Check sheet for the modelled part. Datum: model origin and axes. Units: mm. A direction names the side the tool comes from. Give positions to 0.01 mm unless a question says otherwise; leave off trailing zeros. Write each loop counter-clockwise with the first axis right and the second up, starting at its lowest first coordinate (ties: lowest second). Pieces come first, ordered by that corner, then holes. Notation, with made-up numbers: M 80,8 L 96,8 A16 cw 96,18 Z; hole C 27,4 d8. An arc over 180 degrees is marked long. Use CSV: the item, a comma, the result in double quotes. Start each with the question number.
1. Scan lines: line 1 (Z direction, x = 152.5, y = -0.55); line 2 (Z direction, x = -189.5, y = -0.05); line 3 (X direction, y = -1.05, z = 150.5). Record each from-to range of solid material in increasing order.
2. Access from +Z, -Z, +X, -X, +Y, -Y to the whole of each face (thin tool, end or side, straight path). Record for faces 4 (the face through (311.773, -1.014, 21.597)), 5 (the face through (321.043, -0.986, 13.897)).
3. Mould release check, pull along X, two halves, no side actions. Record for faces 1 (the face through (23, 0, 10)), 2 (the face through (182.02, -0.99, 188.06)), 3 (the face through (173.48, -1.01, 179.63)): +X half, -X half, draft (parallel to the pull), parting line (faces both ways), or undercut.
4. Depth check by flat-ended pin: P1, Ø0.6, axis at x = -54, y = -1, coming from the +Z side. Enter the tip coordinate at first touch or a pass-through.
5. Cross-section at A-A, the plane x = -15. Enter the section's corners in (y, z).
6. Cross-section at C-C, the plane z = 99. Enter the section's corners in (x, y).
7. Cross-section at B-B, the plane y = -0.3. Enter the section's corners in (x, z), and give its area (3 significant figures).
from build123d import *

# Parameters (mm, degrees)
F1_DEPTH = 2
F3_DEPTH = 2
F4_W     = 650
F4_H     = 6
F5_DEPTH = 2


with BuildPart() as f1:
    # F0 (on Front) → F1 (new body)
    with BuildSketch(Plane.XZ):
        Polygon((327.300058, 30.053136), (333.664019, 36.417097), (26.07257, 344.008547), (0, 344.008547), (-26.07257, 344.008547), (-333.664019, 36.417097), (-327.300058, 30.053136), (-332.249806, 25.103389), (-307.146417, 0), (0, 0), (307.146417, 0), (332.249806, 25.103389), align=None)
    extrude(amount=F1_DEPTH)

    # F2 (on face) → F3 (cut)
    with BuildSketch(Plane.XZ.offset(2)):
        Polygon((321.643204, 31.46735), (21.102007, 332.008547), (0, 332.008547), (-21.102007, 332.008547), (-321.643204, 31.46735), (-302.175854, 12), (0, 12), (302.175854, 12), align=None)
    extrude(amount=-F3_DEPTH, mode=Mode.SUBTRACT)

    # F4 (on face) → F5 (cut)
    with BuildSketch(Plane.XZ.offset(2)):
        Rectangle(F4_W, F4_H)
    extrude(amount=-F5_DEPTH, mode=Mode.SUBTRACT)


solid = f1.part
Worked answers:
1,line 1,"z = 3 to 12, 200.61 to 217.58"
1,line 2,"z = 3 to 12, 163.61 to 180.58"
1,line 3,"x = -219.58 to -202.61, 202.61 to 219.58"
2,face 4,"+Y, -Y"
2,face 5,"-Z, +X, +Y, -Y"
3,face 1,"draft"
3,face 2,"+X half"
3,face 3,"undercut"
4,P1,"stops at z = 316.38"
5,outline,"M -2,3 L 0,3 L 0,12 L -2,12 Z; M -2,332.01 L 0,332.01 L 0,344.01 L -2,344.01 Z"
6,outline,"M -271.08,-2 L -254.11,-2 L -254.11,0 L -271.08,0 Z; M 254.11,-2 L 271.08,-2 L 271.08,0 L 254.11,0 Z"
7,outline,"M -333.66,36.42 L -327.3,30.05 L -332.25,25.1 L -310.15,3 L 310.15,3 L 332.25,25.1 L 327.3,30.05 L 333.66,36.42 L 26.07,344.01 L -26.07,344.01 Z; hole M -321.64,31.47 L -302.18,12 L 302.18,12 L 321.64,31.47 L 21.1,332.01 L -21.1,332.01 Z"
7,area,"17,200 mm^2"
